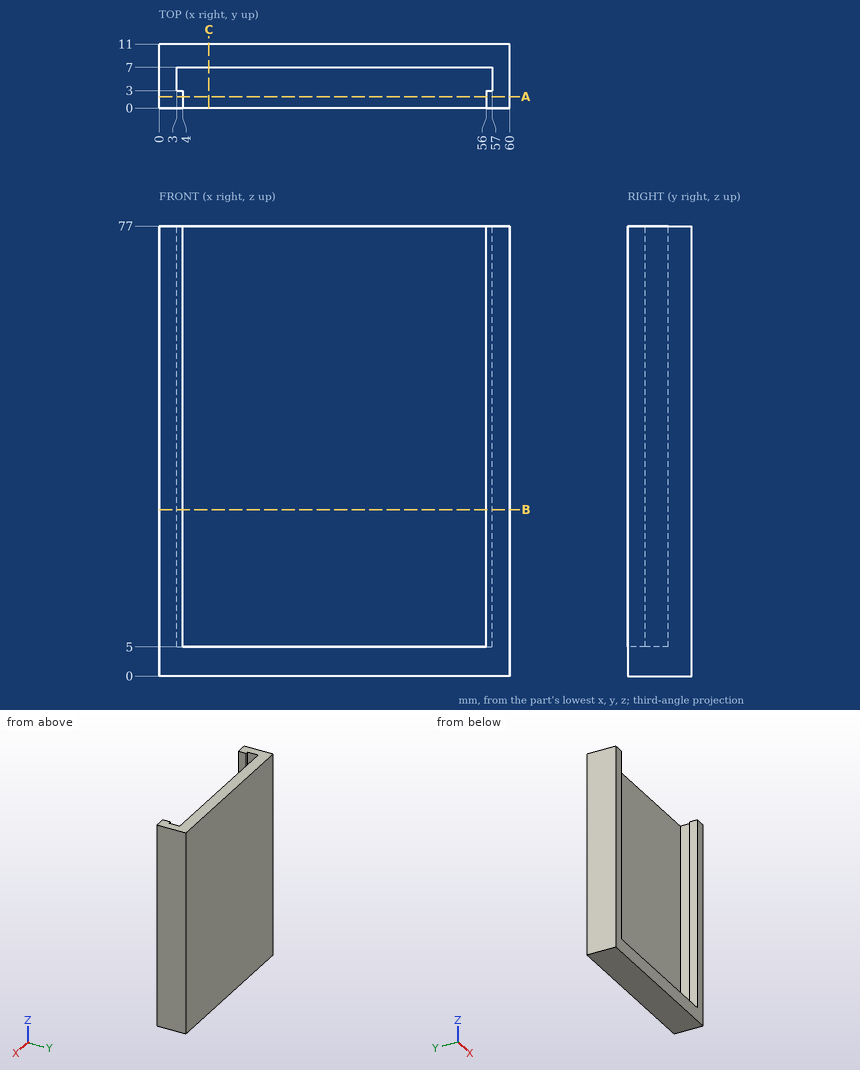
Study the drawing (mm; zero at the part's minimum x, y, z) and answer. Round coordinates to 2 decimals unless told otherwise and drop trailing zeros. Write each loop counter-clockwise with the first axis right and the second up, starting at its lowest first coordinate (ties: lowest second). Pieces come first, ordered by that corner, then holes.
1) A cutting plane is placed at C-C on x = 8.5. Determine the outline of the cut face in (y, z).
2) A cutting plane is placed at A-A on y = 2. Determine the outline of the cut face in (x, z).
3) A cutting plane is placed at B-B on z = 28.5. Determine the outline of the cut face in (x, y).
4) Flat-ended cylindrical pins translate along their axes: P1, Ø4, axis at x = 30.5, y = 4.5, coming from the +Z side; P2, Ø10, axis at x = 22, z = 36.5, coming from the -Y side. Find the tip coordinate at first contact, or state that the pin passes through.
5) Consider probe 1 along X at (y, z) = (2.25, 66); probe 2 along X at (y, z) = (3.25, 72); probe 3 along Z at (x, y) = (19, 1.75). Determine where each line is inside the solid, lowest interval first.
Entries:
1. outline: (0, 0) - (11, 0) - (11, 77) - (7, 77) - (7, 5) - (0, 5) - close
2. outline: (0, 0) - (60, 0) - (60, 77) - (56, 77) - (56, 5) - (4, 5) - (4, 77) - (0, 77) - close
3. outline: (0, 0) - (4, 0) - (4, 3) - (3, 3) - (3, 7) - (57, 7) - (57, 3) - (56, 3) - (56, 0) - (60, 0) - (60, 11) - (0, 11) - close
4. P1: stops at z = 5
4. P2: stops at y = 7
5. probe 1: x = 0 to 4, 56 to 60
5. probe 2: x = 0 to 3, 57 to 60
5. probe 3: z = 0 to 5
